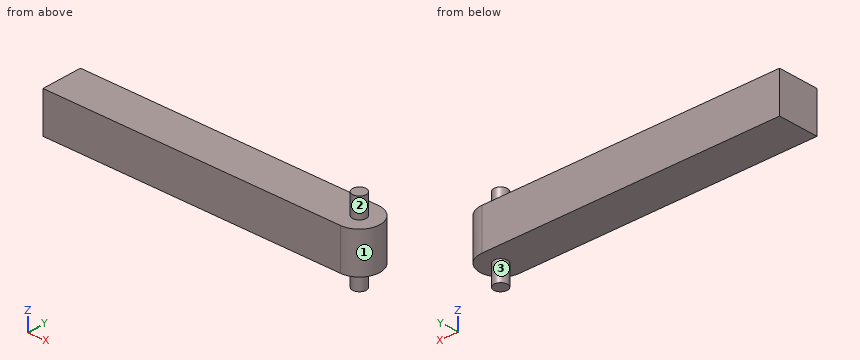
Autodesk Inventor part; units mm, degrees
ref_plane "YZ Plane" through (0, 0, 0) normal (1, 0, 0) x (0, 1, 0)
ref_plane "XZ Plane" through (0, 0, 0) normal (0, 1, 0) x (-1, 0, 0)
ref_plane "XY Plane" through (0, 0, 0) normal (0, 0, 1) x (1, 0, 0)
sketch "Sketch1" plane through (0, 0, 0) normal (0, 0, 1) x (1, 0, 0)
  line L0 (0, 6) -> (47, 6)
  line L1 (56, 0) -> (0, 0)
  line L2 (47, 0) -> (47, 6)
  circle A0 centre (44, 3) radius 1
  line L3 (0, 0) -> (0, 6)
  arc A1 (44, 0) -> (44, 6) centre (44, 3) ccw
  dimension "d26" = 2
  dimension "d29" = 47
  dimension "d30" = 3
  dimension "d31" = 3
  dimension "d32" = 6
extrude "Extrusion1" add sketch "Sketch1" along normal mid plane 6 contours L0 A1 L1 L3 | A0
sketch "Sketch6" plane through (0, 0, 3) normal (0, 0, 1) x (1, 0, 0)
  line L0 (0, 6) -> (47, 6)
  line L1 (47, 0) -> (47, 6)
  circle A0 centre (44, 3) radius 1
  line L2 (0, 0) -> (0, 6)
  arc A1 (44, 0) -> (44, 6) centre (44, 3) ccw
  line L3 (0, 0) -> (44, 0)
  line L4 (44, 6) -> (0, 6)
  dimension "d34" = 2
  dimension "d36" = 3
  dimension "d37" = 3
extrude "Extrusion4" add sketch "Sketch6" along normal blind 3 and the other way blind 9 contours A0
properties part number "Arm"
Work out the finished part from the listing and answer in its coordinate system (mm). Face numbers are marked on the shaded views. A direction names the side the tool comes from. Give positions to 0.01 mm unless a question says otherwise; leave off trailing zeros. Write each loop counter-clockwise with the first axis right and the second up, starting at its lowest first coordinate (ties: lowest second). Pieces come first, ordered by that corner, then holes. Notation, with made-up numbers: (-33.5, 68.25) - (-1.5, 68.25) arc R24 ccw to (-1.5, 104.25) - close; hole circle Ø8 at (-29.75, 37.25). An arc over 180 degrees is marked (long way). Use one line per item in the form item = value.
1. A cutting plane is placed at D-D (y = 0.85). Write down the section's boundary in (x, z), and give its area (3 significant figures).
Filled in:
outline = (0, -3) - (46.09, -3) - (46.09, 3) - (0, 3) - close
area = 277 mm^2
2. A cutting plane is placed at B-B (z = 3.5). Write down the section's boundary in (x, y), and give its area (3 significant figures).
Filled in:
outline = circle Ø2 at (44, 3)
area = 3.14 mm^2
3. A cutting plane is placed at C-C (x = 30). Write down the section's boundary in (y, z), and give its area (3 significant figures).
Filled in:
outline = (0, -3) - (6, -3) - (6, 3) - (0, 3) - close
area = 36.0 mm^2
4. Consider L1, parallel to Z at x = 43.5, y = 5.05; L2, parallel to X at y = 2.95, z = -3.75; L3, parallel to X at y = 0.45, z = -0.75. Determine where each line is inside the solid, lowest interval first.
Filled in:
L1 = -3 to 3
L2 = 43 to 45
L3 = 0 to 45.58
5. For the marked faces 1, 2 and 3, determine the directions among +Z, -Z, +X, -X, +Y, -Y from which every point of the face is accessible in a straight line to the end or side of a thin tool.
Filled in:
face_1 = +Z, -Z, +X
face_2 = +Z
face_3 = -Z
6. Each of these flat-tipped pins is pushed along its axis until it touches: pin 1 Ø1.5 at (x, y) = (19, 1.5) entering from -Z; pin 2 Ø3 at (x, y) = (19.5, 4) entering from +Z. Where does it stop, or does it pass through?
Filled in:
pin_1 = -3
pin_2 = 3
7. A cutting plane is placed at A-A (y = 3). Write down the section's boundary in (x, z).
Filled in:
outline = (0, -3) - (43, -3) - (43, -6) - (45, -6) - (45, -3) - (47, -3) - (47, 3) - (45, 3) - (45, 6) - (43, 6) - (43, 3) - (0, 3) - close
